Can you work these out from the model? Positions are in its coordinate system, mm. Give positions to 0.01 mm unless a question says otherwise; leave off trailing zeros. Write each loop counter-clockwise with the first axis right and the second up, starting at its lowest first coordinate (ties: lowest second). Pieces come first, ordered by that corner, then holes. Notation, with made-up numbers: (76.25, 23) - (107.25, 23) arc R19 ccw to (107.25, 43) - close; hole circle Ø6 at (3.25, -2). An arc over 180 degrees is marked (long way). Return JSON: item names as keys, results as strings. Group by question number.
from build123d import *

# Parameters (mm, degrees)
SKETCH1_R               = 0.8382
BOSS_EXTRUDE1_DEPTH     = 19.05
SKETCH7_R               = 1.8034
CUT_EXTRUDE5_DEPTH      = 2.54
SKETCH8_W               = 2.9464
SKETCH8_H               = 6.35
CUT_EXTRUDE6_DEPTH      = 3.3114
CUT_EXTRUDE6_DEPTH_BACK = 1.635


with BuildPart() as part:
    # Sketch1 → Boss-Extrude1 (new body)
    with BuildSketch(Plane.XY):
        with BuildLine():
            Line((-11.0348776, 1.636724806), (-11.0348776, 2.271724806))
            Line((-11.0348776, 2.271724806), (-4.296180386, 2.271724806))
            ThreePointArc((-4.296180386, 2.271724806), (-2.400761669, 4.41475324), (-3.0846776, 1.636724806))
            Line((-3.0846776, 1.636724806), (-11.0348776, 1.636724806))
        make_face()
        with Locations((-3.0846776, 3.109924806)):
            Circle(SKETCH1_R, mode=Mode.SUBTRACT)
    extrude(amount=BOSS_EXTRUDE1_DEPTH)

    # Sketch7 → Cut-Extrude5 (cut)
    with BuildSketch(Plane(origin=(0, 2.271724806, 0), x_dir=(1, 0, 0), z_dir=(0, 1, 0))):
        with Locations((-7.872478375, -3.9624)):
            Circle(SKETCH7_R)
        with Locations((-7.872478375, -15.0876)):
            Circle(SKETCH7_R)
    extrude(amount=-CUT_EXTRUDE5_DEPTH, mode=Mode.SUBTRACT)

    # Sketch8 → Cut-Extrude6 (cut, two sides)
    with BuildSketch(Plane(origin=(0, 2.271724806, 0), x_dir=(1, 0, 0), z_dir=(0, 1, 0))) as cut_extrude6_sk:
        with Locations((-3.0846776, -9.525)):
            Rectangle(SKETCH8_W, SKETCH8_H)
    extrude(amount=CUT_EXTRUDE6_DEPTH, mode=Mode.SUBTRACT)
    extrude(cut_extrude6_sk.sketch, amount=-CUT_EXTRUDE6_DEPTH_BACK, mode=Mode.SUBTRACT)


solid = part.part
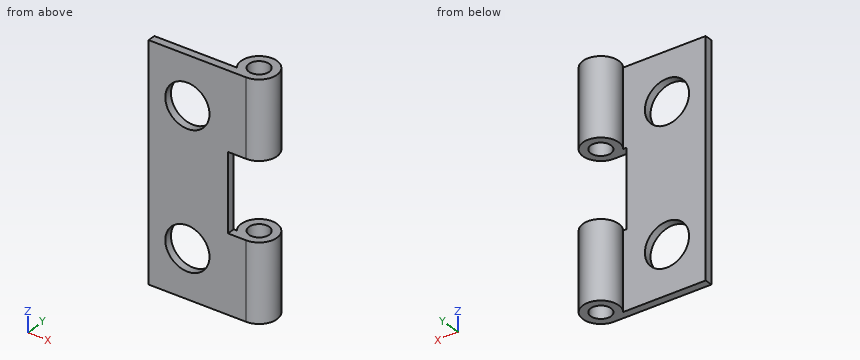
1) Imagine slicing it at C-C, the plane z = 16.5. Write out the boundary of the cut face in (x, y), and give its area (3 significant figures).
2) Will these pins go through, and if not, where does the flat tip stop? pin 1 Ø1.5 at (x, y) = (-9, 4) entering from +Z; pin 2 Ø5.5 at (x, z) = (-9, 12) entering from +Y; pin 3 Ø1.5 at (x, y) = (-3.5, 4) entering from -Z; pin 4 Ø1 at (y, z) = (4, 4.5) entering from -X.
3) Imagine slicing it at A-A, the plane y = 2.8. Write out the boundary of the cut face in (x, z), and give its area (3 significant figures).
4) Imagine slicing it at B-B, the plane x = -2.5. Write out the boundary of the cut face in (y, z), and give its area (3 significant figures).
5) Imagine slicing it at D-D, the plane x = -7. Write out the boundary of the cut face in (y, z).
6) I need wall thicknesses on line 1 along Z through (x, y) = (-4, 3.45); line 2 along Y through (x, z) = (-5.75, 11); line 3 along X through (y, z) = (2.45, 16.25). Which ranges of each line are inside material? Lowest first, please.
Resolved:
{
 "1": {"outline": "(-11.03, 1.64) - (-8.99, 1.64) - (-8.99, 2.27) - (-11.03, 2.27) - close; (-6.75, 1.64) - (-3.08, 1.64) arc R1.47 ccw (long way) to (-4.3, 2.27) - (-6.75, 2.27) - close; hole circle Ø1.68 at (-3.08, 3.11)", "area": "7.70 mm^2"},
 "2": {"pin 1": "through", "pin 2": "y = 2.27", "pin 3": "z = 0", "pin 4": "x = -4.51"},
 "3": {"outline": "(-4.52, 0) - (-3.86, 0) - (-3.86, 6.35) - (-4.52, 6.35) - close; (-4.52, 12.7) - (-3.86, 12.7) - (-3.86, 19.05) - (-4.52, 19.05) - close; (-2.31, 0) - (-1.64, 0) - (-1.64, 6.35) - (-2.31, 6.35) - close; (-2.31, 12.7) - (-1.64, 12.7) - (-1.64, 19.05) - (-2.31, 19.05) - close", "area": "16.8 mm^2"},
 "4": {"outline": "(1.76, 0) - (2.51, 0) - (2.51, 6.35) - (1.76, 6.35) - close; (1.76, 12.7) - (2.51, 12.7) - (2.51, 19.05) - (1.76, 19.05) - close; (3.71, 0) - (4.46, 0) - (4.46, 6.35) - (3.71, 6.35) - close; (3.71, 12.7) - (4.46, 12.7) - (4.46, 19.05) - (3.71, 19.05) - close", "area": "19.1 mm^2"},
 "5": {"outline": "(1.64, 0) - (2.27, 0) - (2.27, 2.38) - (1.64, 2.38) - close; (1.64, 5.54) - (2.27, 5.54) - (2.27, 13.51) - (1.64, 13.51) - close; (1.64, 16.67) - (2.27, 16.67) - (2.27, 19.05) - (1.64, 19.05) - close"},
 "6": {"line 1": "0 to 6.35, 12.7 to 19.05", "line 2": "1.64 to 2.27", "line 3": "-4.4 to -3.6, -2.57 to -1.77"}
}
